Source: CAD feature listing. Evaluate the final solid. Frame: model axes, mm. Round coordinates to 2 decimals unless told otherwise and drop trailing zeros. Order: outer loops, then holes, each group sorted by start corner. A loop starts at its lowest first (then second) coordinate and runs counter-clockwise, first axis right, second up. Notation, with made-up numbers: (75.5, 85.25) -> (99.5, 85.25) arc R21 cw to (99.5, 122.25) -> close; hole circle Ø6 at (29, 78.25). An arc over 180 degrees is marked (long way). Answer as CSV lines item,"result".
Autodesk Inventor part; units mm, degrees
ref_plane "YZ Plane" through (0, 0, 0) normal (1, 0, 0) x (0, 1, 0)
ref_plane "XZ Plane" through (0, 0, 0) normal (0, 1, 0) x (-1, 0, 0)
ref_plane "XY Plane" through (0, 0, 0) normal (0, 0, 1) x (1, 0, 0)
sketch "Sketch1" plane through (0, 0, 0) normal (0, 0, 1) x (1, 0, 0)
  line L0 (75, 110) -> (-75, 110)
  line L1 (-75, 110) -> (-75, -110)
  line L2 (-75, -110) -> (75, -110)
  line L3 (75, -110) -> (75, 110)
  circle A0 centre (0, 0) radius 22.25
  circle A1 centre (0, -26.75) radius 1
  circle A2 centre (0, 26.75) radius 1
  circle A3 centre (108.4721, 5.5003) radius 1.5
  circle A4 centre (70.5, 105) radius 1
  circle A5 centre (-70.5, 105) radius 1
  circle A6 centre (70.5, -105) radius 1
  circle A7 centre (-70.5, -105) radius 1
  dimension "d0" = 150
  dimension "d1" = 220
  dimension "d2" = 44.5
  dimension "d3" = 2
  dimension "d4" = 2
  dimension "d5" = 3
  dimension "d6" = 2
  dimension "d7" = 2
  dimension "d8" = 2
  dimension "d9" = 2
extrude "Extrusion1" add sketch "Sketch1" along normal blind 5 contours L3 L2 L1 L0
sketch "Sketch2" plane through (0, 0, 5) normal (0, 0, 1) x (1, 0, 0)
  line L0 (-34.154, 91.1798) -> (34.154, 91.1798) construction
  line L1 (34.154, 91.1798) -> (34.154, 70.4938) construction
  line L2 (34.154, 70.4938) -> (-34.154, 70.4938) construction
  line L3 (-34.154, 70.4938) -> (-34.154, 91.1798) construction
  point P0 (0, 0)
hole "Hole1" at (71.2413, 25.6886, 5) direction (0, 0, -1) diameter 2 end through all
hole "Hole2" at (-71.9717, 26.0836, 5) direction (0, 0, -1) diameter 2 end through all
hole "Hole3" at (-72.3668, 38.3308, 5) direction (0, 0, -1) diameter 2 end through all
hole "Hole4" at (71.4388, 38.7259, 5) direction (0, 0, -1) diameter 2 end through all
hole "Hole5" at (-71.1816, -25.2755, 5) direction (0, 0, -1) diameter 2 end through all
hole "Hole6" at (71.2413, -27.0533, 5) direction (0, 0, -1) diameter 2 end through all
hole "Hole7" at (71.4388, -41.6709, 5) direction (0, 0, -1) diameter 2 end through all
hole "Hole8" at (-71.3791, -42.2635, 5) direction (0, 0, -1) diameter 2 end through all
properties part number "FrontplatteII"
1. Mould query, pull axis X, two halves, no side actions, for faces 1 (the flat face through (1, 110, 2)), 2 (the flat face through (-75, 2, 2)), 3 (the cylindrical face through (-16.399, -15.038, 2.465)). Classes: released by +X, released by -X, zero draft, split by the parting line, or undercut.
Results below:
face 1,"zero draft"
face 2,"released by -X"
face 3,"undercut"
2. Pin query (flat end, axial travel): pin 1 (2.5 mm diameter, centred on x = -71.18, y = -25.28, fed in from +Z); pin 2 (1.8 mm diameter, centred on x = 71.44, y = 38.73, fed in from +Z). Return the tip coordinate at first contact, or that it passes through.
Results below:
pin 1,"z = 5"
pin 2,"through"
3. Section query B-B on z = 1.1. Give the number of separate pieces and of enclosed holes in the cut face, and give its area (3 significant figures).
Results below:
separate pieces,"1"
enclosed holes,"15"
area,"31,400 mm2"
4. Section query A-A on y = 0. Return loops of the section in (x, z).
Results below:
outline,"(-75, 0) -> (-22.25, 0) -> (-22.25, 5) -> (-75, 5) -> close; (22.25, 0) -> (75, 0) -> (75, 5) -> (22.25, 5) -> close"
5. Line query: L1, parallel to X at y = 105, z = 2.4; L2, parallel to X at y = -27, z = 0.7; L3, parallel to Y at x = 0, z = 3.9. Output: solid intervals per line, ascending. Write a range as [from, to].
Results below:
L1,"[-75, -71.5], [-69.5, 69.5], [71.5, 75]"
L2,"[-75, -0.97], [0.97, 70.24], [72.24, 75]"
L3,"[-110, -27.75], [-25.75, -22.25], [22.25, 25.75], [27.75, 110]"
